Could you check a few things on this model? Use its own coordinates, in mm. A direction names the side the tool comes from. Round coordinates to 2 decimals unless told otherwise and drop trailing zeros. Loops run counter-clockwise (first coordinate to the right, second up) from the corner with the lowest first, then second, coordinate; pieces in that order, holes last.
from build123d import *

# Parameters (mm, degrees)
SKETCH1_W                  = 50.8
SKETCH1_H                  = 63.5
BOSS_EXTRUDE1_DEPTH        = 12.7
F_22_0_22_DIAMETER_HOLE1_D = 22
F_8_32_TAPPED_HOLE1_D      = 3.4544
F_8_32_TAPPED_HOLE1_DEPTH  = 10.668
F_8_32_TAPPED_HOLE1_TIP    = 1.037806461
F_4_CLEARANCE_HOLE1_D      = 2.9464
CIRPATTERN1_COUNT          = 3


with BuildPart() as part:
    # Sketch1 → Boss-Extrude1 (new body)
    with BuildSketch(Plane(origin=(0, 0, 0), x_dir=(0, 0, -1), z_dir=(1, 0, 0))):
        Rectangle(SKETCH1_W, SKETCH1_H)
    extrude(amount=BOSS_EXTRUDE1_DEPTH)

    # Ø22.0 (22) Diameter Hole1 (through all)
    with Locations(Plane(origin=(12.7, 0, 0), x_dir=(0, 0, -1), z_dir=(1, 0, 0))):
        with Locations((0, -12.7)):
            Hole(F_22_0_22_DIAMETER_HOLE1_D / 2)

    # #8-32 Tapped Hole1
    with Locations(Plane(origin=(0, 31.75, 0), x_dir=(1, 0, 0), z_dir=(0, 1, 0))):
        with Locations((6.35, 19.05), (6.35, -19.05), (6.35, 0)):
            Hole(F_8_32_TAPPED_HOLE1_D / 2, depth=F_8_32_TAPPED_HOLE1_DEPTH)
            with Locations((0, 0, -(F_8_32_TAPPED_HOLE1_DEPTH + F_8_32_TAPPED_HOLE1_TIP / 2))):  # 118° drill point
                Cone(0, F_8_32_TAPPED_HOLE1_D / 2, F_8_32_TAPPED_HOLE1_TIP, mode=Mode.SUBTRACT)

    # #4 Clearance Hole1 (through all)
    with Locations(Plane.ZY):
        with Locations((0, 0)):
            f_4_clearance_hole1 = Hole(F_4_CLEARANCE_HOLE1_D / 2)

    # CirPattern1: #4 Clearance Hole1 ×3 about axis
    cirpattern1_axis = Axis((0, -12.7, 0), (1, 0, 0))
    for i in range(1, CIRPATTERN1_COUNT):
        add(f_4_clearance_hole1.rotate(cirpattern1_axis, i * 360 / CIRPATTERN1_COUNT), mode=Mode.SUBTRACT)


solid = part.part
Item 1: For faces 1 (the cylindrical face through (4.703, 26.341, -0.519)), 2 (the flat face through (12.7, 8, 0)), which set-ups out of +Z, -Z, +X, -X, +Y, -Y let a thin tool reach every point of the face, with its end or its side?
Results list:
face 1: +Y
face 2: +Z, -Z, +X, +Y, -Y
Item 2: If we section it at C-C, the plane z = 7: Please give me the cut outline in (x, y).
Results list:
outline: (0, -31.75) - (12.7, -31.75) - (12.7, -21.19) - (0, -21.19) - close; (0, -4.21) - (12.7, -4.21) - (12.7, 31.75) - (0, 31.75) - close
Item 3: If we section it at A-A, the plane y = 0: Please give me the cut outline in (x, z).
Results list:
outline: (0, -25.4) - (12.7, -25.4) - (12.7, -1.47) - (0, -1.47) - close; (0, 1.47) - (12.7, 1.47) - (12.7, 25.4) - (0, 25.4) - close
Item 4: Will this pin go through, and if not, where does the flat tip stop? pin 1 (1 mm diameter, centred on x = 7, z = 18.5, fed in from +Y).
Results list:
pin 1: stops at y = 20.86
Item 5: If we section it at B-B, the plane y = 24: Please give me the cut outline in (x, z), then the cut area to 3 significant figures.
Results list:
outline: (0, -25.4) - (12.7, -25.4) - (12.7, 25.4) - (0, 25.4) - close; hole circle Ø3.45 at (6.35, -19.05); hole circle Ø3.45 at (6.35, 0); hole circle Ø3.45 at (6.35, 19.05)
area: 617 mm2
Item 6: We'd pull the mould along Y, two halves only. Please class faces 3 (the flat face through (6, 0, -25.4)), 4 (the flat face through (9, 31.75, 0)), 5 (the cylindrical face through (6.439, 0.443, -1.405)), 6 (the cylindrical face through (6.439, -17.808, 10.207)): released by +Y, released by -Y, zero draft, split by the parting line, or undercut.
Results list:
face 3: zero draft
face 4: released by +Y
face 5: undercut
face 6: undercut
Item 7: If I drill on line 1 along Z through (x, y) = (6.35, 28.75); line 2 along Y through (x, z) = (3.5, 0); line 3 along Z through (x, y) = (2.5, -9), over which ranges is the centre line in solid material (lowest first)?
Results list:
line 1: z = -25.4 to -20.78, -17.32 to -1.73, 1.73 to 17.32, 20.78 to 25.4
line 2: y = -31.75 to -23.7, -1.7 to -1.47, 1.47 to 31.75
line 3: z = -25.4 to -10.36, 10.36 to 25.4
Item 8: If we section it at D-D, the plane x = 11.25: Please give me the cut outline in (y, z).
Results list:
outline: (-31.75, -25.4) - (31.75, -25.4) - (31.75, 25.4) - (-31.75, 25.4) - close; hole circle Ø22 at (-12.7, 0); hole circle Ø2.95 at (-19.05, -11); hole circle Ø2.95 at (-19.05, 11); hole circle Ø2.95 at (0, 0)
